Design review of the part built by this model. Coordinates are the model's own, in mm. Coordinates: 2 decimals unless noted, no trailing zeros. Loops run counter-clockwise (first coordinate to the right, second up) from the corner with the lowest first, then second, coordinate; pieces in that order, holes last. Notation, with made-up numbers: (-37, 18) -> (6, 18) arc R12 cw to (6, 35) -> close; hole circle Ø6 at (13, 52). An arc over 180 degrees is marked (long way). Use one line per item in the form item = value. Start each with the question number.
1. Consider section A-A (x = 62.5). State the section outline as (y, z) points.
2. Consider section B-B (y = 0). State the section outline as (x, z) points, then the cut area to 3 significant figures.
3. The part is to be moulded in two halves that separate along Y. For faces 1 (the face through (106.506, 0.264, 0.245)), 2 (the face through (55, 12.5, 0)), 3 (the face through (55, 0, 17.5)), say which applies: released by +Y, released by -Y, zero draft, split by the parting line, or undercut.
4. Consider section C-C (z = 5.5). State the section outline as (x, y) points.
5. For pin 1 (3 mm diameter, centred on y = 4.5, z = 9.5, fed in from -X); pin 2 (4 mm diameter, centred on y = -9.5, z = -1, fed in from -X); pin 3 (1 mm diameter, centred on y = -7.5, z = 12.5, fed in from -X), all flat-tipped, find the tip position at first contact; note any pin that passes through.
6. Wall thickness on line 1 (Y direction, x = 62, z = 8); line 2 (X direction, y = -5.5, z = -12); line 3 (Y direction, x = -0.5, z = 12): over which ranges is each line inside the solid? List them lowest first. Write a range as from..to.
7. Consider section D-D (y = -7.5). State the section outline as (x, z) points, then the cut area to 3 significant figures.
Autodesk Inventor part; units mm, degrees
ref_plane "YZ Plane" through (0, 0, 0) normal (1, 0, 0) x (0, 1, 0)
ref_plane "XZ Plane" through (0, 0, 0) normal (0, 1, 0) x (-1, 0, 0)
ref_plane "XY Plane" through (0, 0, 0) normal (0, 0, 1) x (1, 0, 0)
sketch "Sketch1" plane through (0, 0, 0) normal (0, 0, 1) x (1, 0, 0)
  line L0 (0, 12.5) -> (112.5, 12.5)
  arc A0 (112.5, -12.5) -> (112.5, 12.5) centre (112.5, 0) ccw
  line L1 (112.5, -12.5) -> (0, -12.5)
  arc A1 (0, 12.5) -> (0, -12.5) centre (0, 0) ccw
  dimension "d0" = 25
  dimension "d2" = 112.5
extrude "Extrusion1" add sketch "Sketch1" along normal mid plane 35
sketch "Sketch2" plane through (0, 0, 17.5) normal (0, 0, 1) x (1, 0, 0)
  arc A0 (112.5, -12.5) -> (112.5, 12.5) centre (112.5, 0) ccw
  circle A1 centre (112.5, 0) radius 6
  circle A2 centre (62.5, 0) radius 6
  dimension "d5" = 12
  dimension "d7" = 50
extrude "Extrusion2" cut sketch "Sketch2" against normal through all
properties part number "ARM"
Geometry check:
q1.outline = (-12.5, -17.5) -> (-6, -17.5) -> (-6, 17.5) -> (-12.5, 17.5) -> close; (6, -17.5) -> (12.5, -17.5) -> (12.5, 17.5) -> (6, 17.5) -> close
q2.outline = (-12.5, -17.5) -> (56.5, -17.5) -> (56.5, 17.5) -> (-12.5, 17.5) -> close; (68.5, -17.5) -> (106.5, -17.5) -> (106.5, 17.5) -> (68.5, 17.5) -> close; (118.5, -17.5) -> (125, -17.5) -> (125, 17.5) -> (118.5, 17.5) -> close
q2.area = 3,970 mm²
q3.face_1 = undercut
q3.face_2 = released by +Y
q3.face_3 = zero draft
q4.outline = (0, -12.5) -> (112.5, -12.5) arc R12.5 ccw to (112.5, 12.5) -> (0, 12.5) arc R12.5 ccw to start; hole circle Ø12 at (62.5, 0); hole circle Ø12 at (112.5, 0)
q5.pin_1 = -12.13
q5.pin_2 = -10
q5.pin_3 = -10.36
q6.line_1 = -12.5..-5.98, 5.98..12.5
q6.line_2 = -11.22..60.1, 64.9..110.1, 114.9..123.72
q6.line_3 = -12.49..12.49
q7.outline = (-10, -17.5) -> (122.5, -17.5) -> (122.5, 17.5) -> (-10, 17.5) -> close
q7.area = 4,640 mm²
